from build123d import *

# Parameters (mm, degrees)
BOSS_EXTRU_1_DEPTH                                 = 40
ENL_V_MAT_EXTRU_1_DEPTH                            = 43.650205158
ENL_V_MAT_EXTRU_1_DEPTH_BACK                       = 43.650205158
ENL_V_MAT_EXTRU_3_DEPTH                            = 40
CHAMBRAGE_POUR_VIS_T_TE_HEXAGONALE_M31_D           = 3.4
CHAMBRAGE_POUR_VIS_T_TE_HEXAGONALE_M31_CBORE_D     = 4.2
CHAMBRAGE_POUR_VIS_T_TE_HEXAGONALE_M31_CBORE_DEPTH = 3
ESQUISSE6_W                                        = 7.050171065
ESQUISSE6_H                                        = 7.359112957
ENL_V_MAT_EXTRU_4_DEPTH                            = 10
BOSS_EXTRU_2_DEPTH                                 = 50
ESQUISSE9_W                                        = 5
ESQUISSE9_H                                        = 2.5
ENL_V_MAT_EXTRU_5_DEPTH                            = 51.216531143
ESQUISSE11_W                                       = 2
ESQUISSE11_H                                       = 5
ESQUISSE11_W_2                                     = 2.243048
ENL_V_MAT_EXTRU_6_DEPTH                            = 10
ESQUISSE13_W                                       = 10
ESQUISSE13_H                                       = 6.5
ENL_V_MAT_EXTRU_7_DEPTH                            = 6.5
ESQUISSE14_W                                       = 10
ESQUISSE14_H                                       = 6.5
ENL_V_MAT_EXTRU_8_DEPTH                            = 6.5
BOSS_EXTRU_3_DEPTH                                 = 6.5
ESQUISSE15_W                                       = 21
ESQUISSE15_H                                       = 2
ENL_V_MAT_EXTRU_9_DEPTH                            = 5
BOSS_EXTRU_4_DEPTH                                 = 3.6
ESQUISSE17_R                                       = 1.5
BOSS_EXTRU_5_DEPTH                                 = 300


with BuildPart() as part:
    # Esquisse1 → Boss.-Extru.1 (new body)
    with BuildSketch(Plane.XY):
        Polygon((0, -2), (2, 0), (4.8, 0), (4.8, -10.6), (4.43, -11), (5.42, -12.5), (4.43, -14), (1.23, -14), align=None)
    extrude(amount=BOSS_EXTRU_1_DEPTH)

    # Esquisse2 → Enlèv. mat.-Extru.1 (cut, two sides: drawn at the far end of the back side and taken through both)
    with BuildSketch(Plane(origin=(4.8, 0, 0), x_dir=(0, 0, -1), z_dir=(1, 0, 0)).offset(-ENL_V_MAT_EXTRU_1_DEPTH_BACK)):
        Polygon((-37, -14), (-40, -6.3), (-40, -14), align=None)
    extrude(amount=ENL_V_MAT_EXTRU_1_DEPTH + ENL_V_MAT_EXTRU_1_DEPTH_BACK, mode=Mode.SUBTRACT)

    # Esquisse3 → Enlèv. mat.-Extru.3 (cut)
    with BuildSketch(Plane(origin=(0, -6.5, 0), x_dir=(-1, 0, 0), z_dir=(0, 1, 0))):
        Polygon((-5.706792822, 0), (-1.3, 0), (-4.8, 3.75), (-5.706792822, 3.75), align=None)
    extrude(amount=-ENL_V_MAT_EXTRU_3_DEPTH, mode=Mode.SUBTRACT)

    # Chambrage pour vis à tête hexagonale M31 (through all)
    with Locations(Plane(origin=(-0.2, 2.258699511, 74.572212386), x_dir=(0, 0, -1), z_dir=(-1, 0, 0))):
        with Locations((55.572212386, 11.258699511), (45.572212386, 11.258699511)):
            CounterBoreHole(CHAMBRAGE_POUR_VIS_T_TE_HEXAGONALE_M31_D / 2, CHAMBRAGE_POUR_VIS_T_TE_HEXAGONALE_M31_CBORE_D / 2, CHAMBRAGE_POUR_VIS_T_TE_HEXAGONALE_M31_CBORE_DEPTH)

    # Esquisse6 → Enlèv. mat.-Extru.4 (cut)
    with BuildSketch(Plane(origin=(0.694774347, 0, -0.648456057), x_dir=(-0.6823182503600115, 0, -0.7310552682428687), z_dir=(0.7310552682428687, 0, -0.6823182503600115))):
        with Locations((-6.596251813, -11.630248497)):
            Rectangle(ESQUISSE6_W, ESQUISSE6_H)
    extrude(amount=ENL_V_MAT_EXTRU_4_DEPTH, mode=Mode.SUBTRACT)

    # Esquisse7 → Boss.-Extru.2 (add)
    with BuildSketch(Plane.XY.offset(40)):
        Polygon((4.8, -6.5), (24, -6.5), (24, 0), (22.9, 0), (22.9, 4.3), (24.9, 6.2), (22.9, 8.7), (5.9, 8.7), (3.9, 6.2), (5.9, 4.3), (5.9, 0), (4.8, 0), align=None)
    extrude(amount=-BOSS_EXTRU_2_DEPTH)

    # Esquisse8 → Révolution1 (revolve)
    with BuildSketch(Plane(origin=(14.4, 0, 0), x_dir=(0, 0, -1), z_dir=(1, 0, 0))):
        Polygon((-40, 5.2), (-41.3, 4.2), (-41.3, 2.7), (-40, 2.7), align=None)
    revolve(axis=Axis((14.4, 0.7, 31.308149913), (0, 0, 1)))

    # Esquisse9 → Enlèv. mat.-Extru.5 (cut, through all)
    with BuildSketch(Plane(origin=(0, 0, 0), x_dir=(0, 0, -1), z_dir=(1, 0, 0))):
        with Locations((7.5, 7.45)):
            Rectangle(ESQUISSE9_W, ESQUISSE9_H)
    extrude(amount=ENL_V_MAT_EXTRU_5_DEPTH, mode=Mode.SUBTRACT)

    # Esquisse11 → Enlèv. mat.-Extru.6 (cut)
    with BuildSketch(Plane(origin=(0, 0, 0), x_dir=(1, 0, 0), z_dir=(0, 1, 0))):
        with Locations((23.9, 7.5)):
            Rectangle(ESQUISSE11_W, ESQUISSE11_H)
        with Locations((4.778476, 7.5)):
            Rectangle(ESQUISSE11_W_2, ESQUISSE11_H)
    extrude(amount=ENL_V_MAT_EXTRU_6_DEPTH, mode=Mode.SUBTRACT)

    # Esquisse13 → Enlèv. mat.-Extru.7 (cut)
    with BuildSketch(Plane.ZY.offset(-5.9)):
        with Locations((-5, -3.25)):
            Rectangle(ESQUISSE13_W, ESQUISSE13_H)
    extrude(amount=ENL_V_MAT_EXTRU_7_DEPTH, mode=Mode.SUBTRACT)

    # Esquisse14 → Enlèv. mat.-Extru.8 (cut)
    with BuildSketch(Plane(origin=(22.9, 0, 0), x_dir=(0, 0, -1), z_dir=(1, 0, 0))):
        with Locations((5, -3.25)):
            Rectangle(ESQUISSE14_W, ESQUISSE14_H)
    extrude(amount=ENL_V_MAT_EXTRU_8_DEPTH, mode=Mode.SUBTRACT)

    # Esquisse10 → Boss.-Extru.3 (add)
    with BuildSketch(Plane(origin=(0, 6.2, 0), x_dir=(1, 0, 0), z_dir=(0, 1, 0))):
        Polygon((26.9, 5), (-0.1, 5), (-0.1, 16), (2.1, 16), (2.1, 8.5), (24.7, 8.5), (24.7, 16), (26.9, 16), align=None)
    extrude(amount=-BOSS_EXTRU_3_DEPTH)

    # Esquisse15 → Enlèv. mat.-Extru.9 (cut)
    with BuildSketch(Plane.XY.offset(32)):
        with Locations((14.4, 7.7)):
            Rectangle(ESQUISSE15_W, ESQUISSE15_H)
    extrude(amount=-ENL_V_MAT_EXTRU_9_DEPTH, mode=Mode.SUBTRACT)

    # Esquisse16 → Boss.-Extru.4 (add)
    with BuildSketch(Plane(origin=(24, 0, 0), x_dir=(0, 0, -1), z_dir=(1, 0, 0))):
        with BuildLine():
            Line((-7, -6), (-23, -6))
            ThreePointArc((-23, -6), (-24.5, -4.5), (-23, -3))
            Line((-23, -3), (-7, -3))
            ThreePointArc((-7, -3), (-5.5, -4.5), (-7, -6))
        make_face()
    extrude(amount=BOSS_EXTRU_4_DEPTH)

    # Esquisse17 → Boss.-Extru.5 (add)
    with BuildSketch(Plane.XY.offset(40)):
        with Locations((14.4, 0.7)):
            Circle(ESQUISSE17_R)
    extrude(amount=BOSS_EXTRU_5_DEPTH)


solid = part.part
Geometry: final body of the model. Coordinates: model frame, mm. A direction names the side the tool comes from. Coordinates: 2 decimals unless noted, no trailing zeros. Loops run counter-clockwise (first coordinate to the right, second up) from the corner with the lowest first, then second, coordinate; pieces in that order, holes last. Notation, with made-up numbers: (-32.5, 38.5) - (-19.5, 38.5) arc R33 cw to (-19.5, 71.5) - close; hole circle Ø6 at (64, -32.75). An arc over 180 degrees is marked (long way). Put each result on its own line as item: value. Start each with the question number.
Q1. Line query: line 1 (Z direction, x = 4.2, y = -9); line 2 (Y direction, x = 4.3, z = 19); line 3 (Y direction, x = 2.05, z = 19). Output: solid intervals per line, ascending.
Q2. Set-up query: faces 4 (the flat face through (1.6, -0.3, -9.4)), 5 (the flat face through (14, 0, -10)), 6 (the flat face through (14, 6.2, -8)), 7 (the flat face through (14, 3, 41.3)). Return all of +Z, -Z, +X, -X, +Y, -Y with unobstructed straight access to the full face (end or side cutting, diameter ignored); none if empty.
Q3. Cut plane A-A, the plane z = 236. Return loops of the section in (x, y).
Q4. Pin query (flat end, axial travel): pin 1 Ø3 at (x, y) = (13, -4.5) entering from -Z; pin 2 Ø1.3 at (x, y) = (14, 8) entering from -Z; pin 3 Ø4.5 at (x, z) = (3.5, 27) entering from +Y. Return the tip coordinate at first contact, or that it passes through.
Q5. Pull-direction query (X, two-part tool) for faces 1 (the flat face through (2.1, 3, -12)), 2 (the flat face through (3, 3, -5)), 3 (the flat face through (-0.1, 3, -10)); classes: released by +X, released by -X, zero draft, split by the parting line, or undercut.
Filled sheet:
1. line 1: 3.11 to 17.3, 20.7 to 27.3, 30.7 to 38.95
1. line 2: -14 to -10.7, -7.3 to 0, 5.82 to 6.7
1. line 3: -14 to -11.1, -6.9 to 0
2. face 4: -Z, -X, -Y
2. face 5: -Z, +Y, -Y
2. face 6: -Z, +X, -X, +Y
2. face 7: +Z
3. outline: circle Ø3 at (14.4, 0.7)
4. pin 1: z = -10
4. pin 2: z = -5
4. pin 3: y = 8.51
5. face 1: undercut
5. face 2: zero draft
5. face 3: released by -X
